Can you work these out from the model? Positions are in its coordinate system, mm. Face numbers are marked on the shaded views. A direction names the side the tool comes from. Round coordinates to 2 decimals unless told otherwise and drop trailing zeros. Write each loop counter-clockwise with the first axis right and the second up, starting at its lowest first coordinate (ties: lowest second). Pieces come first, ordered by that corner, then holes. Notation, with made-up numbers: (74.25, -39) -> (113.25, -39) arc R24 ccw to (113.25, -13) -> close; hole circle Ø3 at (34, 82.5). An arc over 180 degrees is marked (long way). Write item = value, one per line. Start each with the question number.
1) I'm going to push flat-ended pins straight in: pin 1 (5 mm diameter, centred on y = -9.5, z = 12, fed in from -X); pin 2 (1.5 mm diameter, centred on x = -2, y = 2, fed in from -Z); pin 3 (2.5 mm diameter, centred on x = -18.5, y = -10.5, fed in from +Z); pin 4 (0.9 mm diameter, centred on x = -4.5, y = 3.5, fed in from -Z). Where does each tip first touch, or does it pass through?
2) For the marked faces 1, 2, 3, 4 and 5, which set-ups out of +Z, -Z, +X, -X, +Y, -Y let a thin tool reach every point of the face, with its end or its side?
3) Thinking about a two-plate mould opening in Z: for the marked faces 6, 7, 8 and 9, which applies, +Z half, -Z half, draft (parallel to the pull), parting line (faces both ways), or undercut?
4) Imagine slicing it at D-D, the plane x = -14.5. Please give me the cut outline in (y, z).
5) Imagine slicing it at A-A, the plane y = -3. Please give me the cut outline in (x, z), then the cut area to 3 significant figures.
6) Imagine slicing it at B-B, the plane z = 9.52. Please give me the cut outline in (x, y).
7) Imagine slicing it at C-C, the plane x = -7.5. Please give me the cut outline in (y, z), then the cut area to 3 significant figures.
8) If I drill on line 1 (Y direction, x = -21.1, z = 9.52); line 2 (X direction, y = -8.5, z = 4.25); line 3 (Z direction, x = -2.75, y = 3), over which ranges is the centre line in solid material (lowest first)?
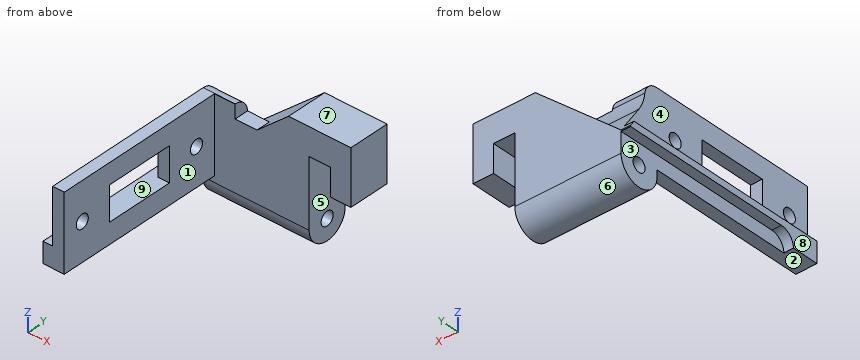
Autodesk Inventor part; units mm, degrees
ref_plane "YZ Plane" through (0, 0, 0) normal (1, 0, 0) x (0, 1, 0)
ref_plane "XZ Plane" through (0, 0, 0) normal (0, 1, 0) x (-1, 0, 0)
ref_plane "XY Plane" through (0, 0, 0) normal (0, 0, 1) x (1, 0, 0)
sketch "Sketch1" plane through (0, 0, 0) normal (0, 1, 0) x (-1, 0, 0)
  line L0 (0, 0) -> (21.6, 0)
  line L1 (21.6, 0) -> (21.6, 17)
  line L2 (21.6, 17) -> (0, 17)
  line L3 (0, 17) -> (0, 0)
  line L4 (6.1, 13) -> (3, 13)
  line L5 (3, 13) -> (3, 0)
  line L6 (3, 0) -> (6.1, 0)
  line L7 (6.1, 0) -> (6.1, 13)
  line L8 (21.6, 17) -> (9.1, 17)
  line L9 (9.1, 17) -> (9.1, 0)
  line L10 (9.1, 0) -> (21.6, 0)
  line L11 (21.6, 0) -> (21.6, 17)
  line L12 (9.1, 17) -> (21.6, 6.2)
  point P0 (21.6, 6.2)
  point P1 (9.1, 17)
  dimension "d1" = 17
  dimension "d2" = 3.1
  dimension "d3" = 3
  dimension "d4" = 3
  dimension "d5" = 6.2
  dimension "d17" = 13
  dimension "d18" = 12.5
extrude "Extrusion1" add sketch "Sketch1" along normal blind 6 contours L3 L2 L9 L0 L7 L4 L5 | L12 L1 L0 L9
sketch "Sketch2" plane through (-21.6, 0, 0) normal (-1, 0, 0) x (0, 0, 1)
  circle A0 centre (3.1, 3) radius 3
  line L0 (0, 0) -> (13, 0)
  line L1 (0, 0) -> (0, 6)
  line L2 (17, 6) -> (0, 6)
  line L3 (0, 0) -> (6.2302, 0)
  line L4 (6.2302, 0) -> (6.2302, 6)
  line L5 (6.2302, 6) -> (0, 6)
  line L6 (0, 6) -> (0, 0)
  circle A1 centre (3.1, 3) radius 1
  point P0 (3.1, 6)
  point P1 (3.1, 0)
  dimension "d8" = 3.1
  dimension "d9" = 2
extrude "Extrusion2" cut sketch "Sketch2" against normal up to surface (18.6 mm away) contours A0 L0 L1 L2 | A1
sketch "Sketch3" plane through (0, 6, 0) normal (0, 1, 0) x (1, 0, 0)
  line L0 (-3, 0) -> (-3, -13)
  line L1 (0, 0) -> (-3, 0)
  line L2 (-3, -9) -> (0, -9)
  line L3 (0, -9) -> (0, 0)
  line L4 (0, 0) -> (-3, 0)
  line L5 (-3, 0) -> (-3, -9)
  line L6 (-3, -13) -> (-6.1, -13)
  line L7 (-9.1, -17) -> (0, -17)
  dimension "d13" = 8
extrude "Extrusion3" cut sketch "Sketch3" against normal blind 10
sketch "Sketch4" plane through (-21.6, 0, 6.2) normal (-1, 0, 0) x (0, 0, 1)
  line L0 (-2.18, -25) -> (8.82, -25)
  line L1 (8.82, -25) -> (8.82, 0)
  line L2 (8.82, 0) -> (-2.18, 0)
  line L3 (-2.18, 0) -> (-2.18, -25)
  circle A0 centre (-3.1, 3) radius 1
  line L4 (0, 0) -> (10.8, 0)
  line L5 (0, 0) -> (0, 6)
  line L6 (8.82, 0) -> (0, 6)
  circle A1 centre (3.32, -22) radius 1
  circle A2 centre (3.32, -3) radius 1
  line L7 (0.82, -17.5) -> (5.82, -17.5)
  line L8 (5.82, -17.5) -> (5.82, -7.5)
  line L9 (5.82, -7.5) -> (0.82, -7.5)
  line L10 (0.82, -7.5) -> (0.82, -17.5)
  point P0 (-6.2, 0)
  dimension "d19" = 0.92
  dimension "d20" = 0
  dimension "d21" = 25
  dimension "d22" = 11
  dimension "d23" = 5.5
  dimension "d24" = 5.5
  dimension "d25" = 5
  dimension "d26" = 10
  dimension "d27" = 7.5
  dimension "d28" = 3
  dimension "d29" = 2
  dimension "d30" = 2
  dimension "d51" = 19
  dimension "d52" = 3
extrude "Extrusion4" add sketch "Sketch4" against normal blind 1.7 contours L3 L2 L1 L0 | L2 L5 L6
sketch "Sketch6" plane through (0, 0, 0) normal (0, -1, 0) x (1, 0, 0)
  line L0 (-19.9, 15.02) -> (-19.9, 4.02)
  line L1 (-19.9, 4.02) -> (-7.9, 4.02)
  line L2 (-7.9, 4.02) -> (-7.9, 15.02)
  line L3 (-7.9, 15.02) -> (-19.9, 15.02)
  line L4 (-19.9, 15.02) -> (-19.9, 4.02)
  line L5 (-12.9, 4.02) -> (-10.3572, 4.02)
  line L6 (-10.3572, 4.02) -> (-10.3572, 15.02)
  line L7 (-10.3572, 15.02) -> (-12.9, 15.02)
  line L8 (-12.9, 15.02) -> (-12.9, 4.02)
  line L9 (-12.9, 15.02) -> (-16.9, 15.02)
  line L10 (-16.9, 15.02) -> (-16.9, 13.02)
  line L11 (-16.9, 13.02) -> (-12.9, 13.02)
  line L12 (-12.9, 13.02) -> (-12.9, 15.02)
  line L13 (-21.6, 15.02) -> (-21.6, 6.2)
  line L14 (-19.9, 4.02) -> (-21.6, 4.02)
  line L15 (-21.6, 4.02) -> (-21.6, 15.02)
  line L16 (-21.6, 15.02) -> (-19.9, 15.02)
  line L17 (-19.9, 15.02) -> (-19.9, 4.02)
  point P0 (0, 0)
  dimension "d33" = 12
  dimension "d34" = 7
  dimension "d35" = 4
  dimension "d36" = 2
extrude "Extrusion5" add sketch "Sketch6" against normal blind 2 contours L3 L10 L11 L8 L1 L0 | L0 L14 L15 L13 L16
sketch "Sketch7" plane through (-21.6, 3, 3.1) normal (-1, 0, 0) x (0, 0, 1)
  line L0 (8.98, -1) -> (3.1, 3)
  line L1 (8.98, -1) -> (3.1, -1)
  line L2 (3.1, -1) -> (3.1, 3)
  line L3 (3.1, 3) -> (8.98, 3)
  line L4 (8.98, 3) -> (8.98, -1)
  line L5 (0, 3) -> (3.1, 3)
  line L6 (3.1, 3) -> (8.98, -1)
  point P0 (-3.1, -3)
extrude "Extrusion6" add sketch "Sketch7" against normal blind 9 contours L1 L2 L0
sketch "Sketch8" plane through (-21.6, 3, 3.1) normal (-1, 0, 0) x (0, 0, 1)
  line L0 (-9.7709, -24.08) -> (2.92, -24.08)
  line L1 (2.92, -24.08) -> (2.92, 6.3077)
  line L2 (2.92, 6.3077) -> (-9.7709, 6.3077)
  line L3 (-9.7709, 6.3077) -> (-9.7709, -24.08)
  line L4 (11.92, -28) -> (11.92, -1)
  line L5 (0.92, -28) -> (11.92, -28)
  line L6 (0.92, -3) -> (0.92, -28)
  line L7 (3.1, 3) -> (8.98, -1)
  line L8 (0.92, -28) -> (3.92, -28)
  line L9 (3.92, -28) -> (3.92, 2.4422)
  line L10 (3.92, 2.4422) -> (0.92, 2.4422)
  line L11 (0.92, 2.4422) -> (0.92, -28)
  line L12 (3.92, -20.5) -> (3.92, -10.5)
  line L13 (2.92, 2.4422) -> (2.92, 3)
  line L14 (3.1, 3) -> (13.9, 3)
  line L15 (2.92, 2.4422) -> (3.92, 2.4422)
  line L16 (3.92, 2.4422) -> (3.92, 3)
  line L17 (3.92, 3) -> (2.92, 3)
  line L18 (2.92, 3) -> (2.92, 2.4422)
  line L19 (3.92, 2.4422) -> (3.1, 3)
  point P0 (-3.1, -3)
  point P1 (0.92, -24.08)
  point P2 (3.92, -28)
  point P3 (2.92, 3)
  dimension "d41" = 9
  dimension "d42" = 3.92
  dimension "d43" = 10.691
  dimension "d44" = 0
  dimension "d45" = 0
extrude "Extrusion7" add sketch "Sketch8" along normal blind 1.4 contours L0 L1 L10 L9 L5 L6 | L1 L17 L7 L10
fillet "Fillet1" radius 2 1 edges at (-22.3, -21.08, 6.02)
fillet "Fillet2" radius 6 1 edges at (-18.1972, 2, 12.08)
fillet "Fillet3" radius 2 1 edges at (-19.25, 2, 15.02)
equation "\"d23\" = 0.5 * d22"
equation "\"d24\" = 0.5 * d22"
equation "\"d27\" = -0.5 * d26 + 0.5 * d21"
equation "\"d28\" = -0.5 * d25 + 0.5 * d22"
equation "\"d52\" = -0.5 * d51 + 0.5 * d21"
properties part number "Pi3B_spacer_R_switch2"
Reported:
q1.pin_1 = -21.6
q1.pin_2 = 9
q1.pin_3 = through
q1.pin_4 = 13
q2.face_1 = +Z, -Z, +X, -Y
q2.face_2 = -Z, +X, -X, -Y
q2.face_3 = -Z, -X, +Y
q2.face_4 = +Z, -X, +Y, -Y
q2.face_5 = -Z, +Y, -Y
q3.face_6 = -Z half
q3.face_7 = +Z half
q3.face_8 = draft
q3.face_9 = undercut
q4.outline = (0, 3.1) arc R3 ccw to (6, 3.1) -> (6, 12.33) -> (2.22, 12.33) arc R6 cw to (2.07, 13.02) -> (0, 13.02) -> close; hole circle Ø2 at (3, 3.1)
q5.outline = (-23, 6.02) -> (-21.6, 6.02) -> (-21.6, 4.02) -> (-19.9, 4.02) -> (-19.9, 8.52) -> (-21.6, 8.52) -> (-21.6, 7.02) -> (-23, 7.02) -> close; (-21.6, 10.52) -> (-19.9, 10.52) -> (-19.9, 15.02) -> (-21.6, 15.02) -> close
q5.area = 16.7 mm²
q6.outline = (-21.6, -25) -> (-19.9, -25) -> (-19.9, -23) -> (-21.6, -23) -> close; (-21.6, -21) -> (-19.9, -21) -> (-19.9, -17.5) -> (-21.6, -17.5) -> close; (-21.6, -7.5) -> (-19.9, -7.5) -> (-19.9, -4) -> (-21.6, -4) -> close; (-21.6, -2) -> (-19.9, -2) -> (-19.9, 0) -> (-6.1, 0) -> (-6.1, 6) -> (-17.76, 6) -> (-17.76, 3.74) -> (-21.6, 3.74) -> close; (-3, 0) -> (0, 0) -> (0, 6) -> (-3, 6) -> close
q7.outline = (0, 3.1) arc R3 ccw to (6, 3.1) -> (6, 17) -> (0, 17) -> close; hole circle Ø2 at (3, 3.1)
q7.area = 94.4 mm²
q8.line_1 = -25 to -23, -21 to -17.5, -7.5 to -4, -2 to 3.74
q8.line_2 = -21.6 to -19.9
q8.line_3 = 9 to 17
